Geometry: final body of the model. Coordinates: model frame, mm. A direction names the side the tool comes from. Give positions to 0.01 mm unless a question says otherwise; leave off trailing zeros. Loops run counter-clockwise (first coordinate to the right, second up) from the corner with the lowest first, then second, coordinate; pieces in that order, holes last. Notation, with made-up numbers: (52, -35.5) - (56, -35.5) arc R10 cw to (56, -19.5) - close; hole circle Ø10 at (-15.5, -19.5). An arc over 180 degrees is marked (long way). Answer in a Markdown table with one row per item.
from build123d import *

# Parameters (mm, degrees)
CROQUIS1_W              = 96.8
CROQUIS1_H              = 40.5
SALIENTE_EXTRUIR1_DEPTH = 2
CROQUIS4_W              = 76.8
CROQUIS4_H              = 40.5
CROQUIS4_W_2            = 72.8
CROQUIS4_H_2            = 36.5
SALIENTE_EXTRUIR6_DEPTH = 33
CORTAR_EXTRUIR2_START   = 10
CROQUIS2_W              = 15
CROQUIS2_H              = 2
CORTAR_EXTRUIR2_DEPTH   = 12
CORTAR_EXTRUIR4_DEPTH   = 33
CORTAR_EXTRUIR5_DEPTH   = 96.756474977
CROQUIS7_R              = 2
CORTAR_EXTRUIR6_DEPTH   = 12
CROQUIS8_W              = 10
CROQUIS8_H              = 3
SALIENTE_EXTRUIR7_DEPTH = 10
SALIENTE_EXTRUIR9_DEPTH = 9.340280327
CROQUIS9_W              = 10
CROQUIS9_H              = 8
SALIENTE_EXTRUIR8_DEPTH = 33
CROQUIS10_R             = 1.25
CORTAR_EXTRUIR7_DEPTH   = 10
CORTAR_EXTRUIR8_REACH   = 74.165
CROQUIS11_R             = 1.25


with BuildPart() as part:
    # Croquis1 → Saliente-Extruir1 (new body)
    with BuildSketch(Plane(origin=(0, 0, 0), x_dir=(1, 0, 0), z_dir=(0, 1, 0))):
        Rectangle(CROQUIS1_W, CROQUIS1_H)
    extrude(amount=SALIENTE_EXTRUIR1_DEPTH)

    # Croquis4 → Saliente-Extruir6 (add)
    with BuildSketch(Plane(origin=(0, 2, 0), x_dir=(1, 0, 0), z_dir=(0, 1, 0))):
        Rectangle(CROQUIS4_W, CROQUIS4_H)
        Rectangle(CROQUIS4_W_2, CROQUIS4_H_2, mode=Mode.SUBTRACT)
    extrude(amount=SALIENTE_EXTRUIR6_DEPTH)

    # Croquis2 → Cortar-Extruir2 (cut)
    with BuildSketch(Plane(origin=(0, 2, 0), x_dir=(1, 0, 0), z_dir=(0, 1, 0)).offset(CORTAR_EXTRUIR2_START)):
        with Locations((-40.9, -19.25)):
            Rectangle(CROQUIS2_W, CROQUIS2_H)
        with Locations((40.9, -19.25)):
            Rectangle(CROQUIS2_W, CROQUIS2_H)
    extrude(amount=-CORTAR_EXTRUIR2_DEPTH, mode=Mode.SUBTRACT)

    # Croquis6 → Cortar-Extruir4 (cut)
    with BuildSketch(Plane(origin=(0, 35, 0), x_dir=(1, 0, 0), z_dir=(0, 1, 0))):
        Polygon((36.4, 18.25), (-36.4, 18.25), (-36.4, 10.909719673), (-38.4, 10.909719673), (-38.4, 20.25), (36.4, 20.25), align=None)
    extrude(amount=-CORTAR_EXTRUIR4_DEPTH, mode=Mode.SUBTRACT)

    # Croquis5 → Cortar-Extruir5 (cut, through all)
    with BuildSketch(Plane(origin=(38.4, 0, 0), x_dir=(0, 0, -1), z_dir=(1, 0, 0))):
        Polygon((1.75, 35), (20.25, 16.5), (20.25, 35), align=None)
    extrude(amount=-CORTAR_EXTRUIR5_DEPTH, mode=Mode.SUBTRACT)

    # Croquis7 → Cortar-Extruir6 (cut)
    with BuildSketch(Plane(origin=(0, 2, 0), x_dir=(1, 0, 0), z_dir=(0, 1, 0))):
        with Locations(Location((42.4, 7.25, 0), (0, 0, 270))):
            Circle(CROQUIS7_R)
        with Locations(Location((42.4, -5.75, 0), (0, 0, 270))):
            Circle(CROQUIS7_R)
        with Locations(Location((-42.9, 5.25, 0), (0, 0, 270))):
            Circle(CROQUIS7_R)
        with Locations(Location((-42.9, -7.75, 0), (0, 0, 270))):
            Circle(CROQUIS7_R)
    extrude(amount=-CORTAR_EXTRUIR6_DEPTH, mode=Mode.SUBTRACT)

    # Croquis8 → Saliente-Extruir7 (add)
    with BuildSketch(Plane(origin=(0, 2, 0), x_dir=(1, 0, 0), z_dir=(0, 1, 0))):
        with Locations((43.4, 18.75)):
            Rectangle(CROQUIS8_W, CROQUIS8_H)
        with Locations((-43.4, 9.409719673)):
            Rectangle(CROQUIS8_W, CROQUIS8_H)
    extrude(amount=SALIENTE_EXTRUIR7_DEPTH)

    # Croquis13 → Saliente-Extruir9 (add)
    with BuildSketch(Plane(origin=(0, 0, -10.909719673), x_dir=(-1, 0, 0), z_dir=(0, 0, -1))):
        with BuildLine():
            Line((45.9, 2), (40.9, 2))
            Line((40.9, 2), (40.9, 9))
            ThreePointArc((40.9, 9), (43.4, 11.5), (45.9, 9))
            Line((45.9, 9), (45.9, 2))
        make_face()
    extrude(amount=SALIENTE_EXTRUIR9_DEPTH)

    # Croquis9 → Saliente-Extruir8 (add)
    with BuildSketch(Plane(origin=(0, 2, 0), x_dir=(1, 0, 0), z_dir=(0, 1, 0))):
        with Locations((-43.4, -14.25)):
            Rectangle(CROQUIS9_W, CROQUIS9_H)
        with Locations((43.4, -14.25)):
            Rectangle(CROQUIS9_W, CROQUIS9_H)
    extrude(amount=SALIENTE_EXTRUIR8_DEPTH)

    # Croquis10 → Cortar-Extruir7 (cut)
    with BuildSketch(Plane(origin=(0, 35, 0), x_dir=(1, 0, 0), z_dir=(0, 1, 0))):
        with Locations(Location((-43.4, -14.25, 0), (0, 0, 270))):
            Circle(CROQUIS10_R)
        with Locations(Location((43.4, -14.25, 0), (0, 0, 270))):
            Circle(CROQUIS10_R)
    extrude(amount=-CORTAR_EXTRUIR7_DEPTH, mode=Mode.SUBTRACT)

    # Cortar-Extruir8: up to this face of the body (flat: up to its plane)
    cortar_extruir8_end = Plane(part.part.faces().sort_by_distance((-43.4, 7, -7.909719673))[0])
    # Croquis11 → Cortar-Extruir8 (cut, up to the picked face)
    with BuildSketch(Plane(origin=(0, 0, -20.25), x_dir=(-1, 0, 0), z_dir=(0, 0, -1)), mode=Mode.PRIVATE) as cortar_extruir8_sk1:
        with Locations((-43.4, 7)):
            Circle(CROQUIS11_R)
    cortar_extruir8_tool1 = split(extrude(cortar_extruir8_sk1.sketch, amount=-CORTAR_EXTRUIR8_REACH, mode=Mode.PRIVATE), bisect_by=cortar_extruir8_end, keep=Keep.BOTH, mode=Mode.PRIVATE)
    # Croquis11 → Cortar-Extruir8 (cut, up to the picked face)
    with BuildSketch(Plane(origin=(0, 0, -20.25), x_dir=(-1, 0, 0), z_dir=(0, 0, -1)), mode=Mode.PRIVATE) as cortar_extruir8_sk2:
        with Locations((43.4, 7)):
            Circle(CROQUIS11_R)
    cortar_extruir8_tool2 = split(extrude(cortar_extruir8_sk2.sketch, amount=-CORTAR_EXTRUIR8_REACH, mode=Mode.PRIVATE), bisect_by=cortar_extruir8_end, keep=Keep.BOTH, mode=Mode.PRIVATE)
    add(cortar_extruir8_tool1.solids().sort_by(Axis((43.4, 7, -20.25), (0, 0, 1)))[0], mode=Mode.SUBTRACT)
    add(cortar_extruir8_tool2.solids().sort_by(Axis((-43.4, 7, -20.25), (0, 0, 1)))[0], mode=Mode.SUBTRACT)


solid = part.part
Q1. Cut plane D-D (x = -16.5). Output: boundary loops of the cut face in (y, z), and give its area (3 significant figures).
Check values:
| item | result |
|---|---|
| outline | (0, -20.25) - (2, -20.25) - (2, 18.25) - (35, 18.25) - (35, 20.25) - (0, 20.25) - close |
| area | 147 mm² |
Q2. First-contact query: pin 1 (4 mm diameter, centred on y = 11, z = 0, fed in from -X); pin 2 (8 mm diameter, centred on x = 44, z = -2, fed in from +Y); pin 3 (7.5 mm diameter, centred on y = 6.5, z = -15, fed in from +X); pin 4 (9 mm diameter, centred on y = 23.5, z = -12, fed in from +X). Flat tips, straight axial feed; report the tip coordinate or a pass-through.
Check values:
| item | result |
|---|---|
| pin 1 | x = -38.4 |
| pin 2 | y = 2 |
| pin 3 | x = 48.4 |
| pin 4 | x = 38.4 |
Q3. Cut plane A-A (y = 14.5). Output: boundary loops of the cut face in (x, z).
Check values:
| item | result |
|---|---|
| outline | (-48.4, 10.25) - (-38.4, 10.25) - (-38.4, -10.91) - (-36.4, -10.91) - (-36.4, 18.25) - (36.4, 18.25) - (36.4, -20.25) - (38.4, -20.25) - (38.4, 10.25) - (48.4, 10.25) - (48.4, 18.25) - (38.4, 18.25) - (38.4, 20.25) - (-38.4, 20.25) - (-38.4, 18.25) - (-48.4, 18.25) - close |
Q4. Reachability of faces 1 (the flat face through (36.4, 19, -1)), 2 (the flat face through (-36, 12, 19)), 3 (the cylindrical face through (-44.62, 30.07, 13.98)) from +Z, -Z, +X, -X, +Y, -Y: full face, straight path, thin tool, end or side. Return the list, or none.
Check values:
| item | result |
|---|---|
| face 1 | -Z, +Y |
| face 2 | +Z, -X, -Y |
| face 3 | +Y |
Q5. Cut plane B-B (z = -0.5). Output: boundary loops of the cut face in (x, y), and give its area (3 significant figures).
Check values:
| item | result |
|---|---|
| outline | (-48.4, 0) - (48.4, 0) - (48.4, 2) - (38.4, 2) - (38.4, 35) - (36.4, 35) - (36.4, 2) - (-36.4, 2) - (-36.4, 35) - (-38.4, 35) - (-38.4, 2) - (-48.4, 2) - close |
| area | 326 mm² |
Q6. Material intervals for line 1 along X through (y, z) = (5.5, 17.5); line 2 along Y through (x, z) = (43.4, -19.5); line 3 along X through (y, z) = (9, 8), sorted ascending.
Check values:
| item | result |
|---|---|
| line 1 | -48.4 to -36.4, 36.4 to 48.4 |
| line 2 | 0 to 5.75, 8.25 to 12 |
| line 3 | -38.4 to -36.4, 36.4 to 38.4 |
Q7. Draft query along X for faces 4 (the flat face through (42, 18, 18.25)), 5 (the cylindrical face through (-43.3, 11.5, -15.5)), 6 (the flat face through (33.4, 6, 19)). Return one class per face: pulls with the +X half, pulls with the -X half, needs draft (parallel to the pull), parting line crosses it, or undercut.
Check values:
| item | result |
|---|---|
| face 4 | needs draft |
| face 5 | undercut |
| face 6 | pulls with the +X half |
Q8. Cut plane C-C (x = 43.4). Output: boundary loops of the cut face in (y, z).
Check values:
| item | result |
|---|---|
| outline | (0, -20.25) - (5.75, -20.25) - (5.75, -17.25) - (2, -17.25) - (2, -8.98) - (0, -8.98) - close; (0, -5.52) - (2, -5.52) - (2, 4.02) - (0, 4.02) - close; (0, 7.48) - (2, 7.48) - (2, 10.25) - (35, 10.25) - (35, 13) - (25, 13) - (25, 15.5) - (35, 15.5) - (35, 18.25) - (0, 18.25) - close; (8.25, -20.25) - (12, -20.25) - (12, -17.25) - (8.25, -17.25) - close |
